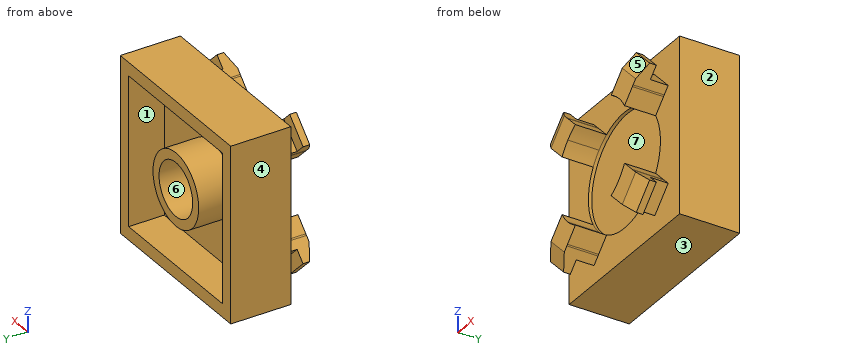
from build123d import *

# Parameters (mm, degrees)
SKETCH2_W            = 15.8
SKETCH2_H            = 15.8
BOSS_EXTRUDE2_DEPTH  = 5.4
SKETCH4_W            = 13.4
SKETCH4_H            = 13.4
CUT_EXTRUDE1_DEPTH   = 3.2
SKETCH7_R            = 3.265
SKETCH7_R_2          = 2.4
BOSS_EXTRUDE5_DEPTH  = 3.2
SKETCH8_R            = 5.15
CUT_EXTRUDE2_DEPTH   = 0.3
BOSS_EXTRUDE8_DEPTH  = 2.8
SKETCH27_W           = 2.7
SKETCH27_H           = 1.2
BOSS_EXTRUDE10_DEPTH = 1.2
CUT_EXTRUDE3_DEPTH   = 2.7
CIRPATTERN1_COUNT    = 4


with BuildPart() as part:
    # Sketch2 → Boss-Extrude2 (new body)
    with BuildSketch(Plane(origin=(0, 0, 0), x_dir=(1, 0, 0), z_dir=(0, 1, 0))):
        with Locations((7.9, 7.9)):
            Rectangle(SKETCH2_W, SKETCH2_H)
    extrude(amount=-BOSS_EXTRUDE2_DEPTH)

    # Sketch4 → Cut-Extrude1 (cut)
    with BuildSketch(Plane(origin=(0, 0, 0), x_dir=(1, 0, 0), z_dir=(0, 1, 0))):
        with Locations((7.9, 7.9)):
            Rectangle(SKETCH4_W, SKETCH4_H)
    extrude(amount=-CUT_EXTRUDE1_DEPTH, mode=Mode.SUBTRACT)

    # Sketch7 → Boss-Extrude5 (add)
    with BuildSketch(Plane(origin=(0, -3.2, 0), x_dir=(1, 0, 0), z_dir=(0, 1, 0))):
        with Locations((7.85, 7.85)):
            Circle(SKETCH7_R)
        with Locations((7.85, 7.85)):
            Circle(SKETCH7_R_2, mode=Mode.SUBTRACT)
    extrude(amount=BOSS_EXTRUDE5_DEPTH)

    # Sketch8 → Cut-Extrude2 (cut)
    with BuildSketch(Plane(origin=(0, -5.4, 0), x_dir=(-1, 0, 0), z_dir=(0, -1, 0))):
        with Locations((-7.9, 7.9)):
            Circle(SKETCH8_R)
    extrude(amount=-CUT_EXTRUDE2_DEPTH, mode=Mode.SUBTRACT)

    # Sketch11 → Boss-Extrude8 (add)
    with BuildSketch(Plane.XZ.offset(5.4)):
        Polygon((11.683021279, -2.207790411), (12.637615434, -3.162384566), (13.203300859, -2.596699141), (12.248706704, -1.642104986), align=None)
        with BuildLine():
            ThreePointArc((11.585853022, -2.304958669), (12.133497372, -2.706975833), (12.637615434, -3.162384566))
            Line((12.637615434, -3.162384566), (11.683021279, -2.207790411))
            Line((11.683021279, -2.207790411), (11.585853022, -2.304958669))
        make_face()
        with BuildLine():
            ThreePointArc((10.459662524, -3.431149167), (11.028098464, -3.808851017), (11.541599923, -4.258400077))
            Line((11.541599923, -4.258400077), (12.637615434, -3.162384566))
            ThreePointArc((12.637615434, -3.162384566), (12.133497372, -2.706975833), (11.585853022, -2.304958669))
            Line((11.585853022, -2.304958669), (10.459662524, -3.431149167))
        make_face()
        with BuildLine():
            Line((12.637615434, -3.162384566), (11.541599923, -4.258400077))
            ThreePointArc((11.541599923, -4.258400077), (11.991148983, -4.771901536), (12.368850833, -5.340337476))
            Line((12.368850833, -5.340337476), (13.495041331, -4.214146978))
            ThreePointArc((13.495041331, -4.214146978), (13.093024167, -3.666502628), (12.637615434, -3.162384566))
        make_face()
        with BuildLine():
            Line((13.592209589, -4.116978721), (12.637615434, -3.162384566))
            ThreePointArc((12.637615434, -3.162384566), (13.093024167, -3.666502628), (13.495041331, -4.214146978))
            Line((13.495041331, -4.214146978), (13.592209589, -4.116978721))
        make_face()
        Polygon((13.203300859, -2.596699141), (12.637615434, -3.162384566), (13.592209589, -4.116978721), (14.157895014, -3.551293296), align=None)
    boss_extrude8 = extrude(amount=BOSS_EXTRUDE8_DEPTH)

    # Sketch27 → Boss-Extrude10 (add)
    with BuildSketch(Plane(origin=(5.303300859, 0, 5.303300859), x_dir=(0.707106781, 0, -0.707106781), z_dir=(0.707106781, 0, 0.707106781))):
        with Locations((11.172287143, -7.6)):
            Rectangle(SKETCH27_W, SKETCH27_H)
    boss_extrude10 = extrude(amount=BOSS_EXTRUDE10_DEPTH)

    # Sketch28 → Cut-Extrude3 (cut)
    with BuildSketch(Plane(origin=(6.945405845, 0, -6.945405845), x_dir=(0.707106781, 0, 0.707106781), z_dir=(-0.707106781, 0, 0.707106781))):
        Polygon((8.7, -7.6), (7.215606324, -8.2), (8.7, -8.2), align=None)
    cut_extrude3 = extrude(amount=-CUT_EXTRUDE3_DEPTH, mode=Mode.SUBTRACT)

    # CirPattern1: Boss-Extrude8, Boss-Extrude10, Cut-Extrude3 ×4 about axis
    cirpattern1_axis = Axis((7.9, 0, -7.9), (0, 1, 0))
    for i in range(1, CIRPATTERN1_COUNT):
        add(boss_extrude8.rotate(cirpattern1_axis, i * 360 / CIRPATTERN1_COUNT))
        add(boss_extrude10.rotate(cirpattern1_axis, i * 360 / CIRPATTERN1_COUNT))
        add(cut_extrude3.rotate(cirpattern1_axis, i * 360 / CIRPATTERN1_COUNT), mode=Mode.SUBTRACT)


solid = part.part
Geometry: final body of the model. Coordinates: model frame, mm. Face numbers are marked on the shaded views. A direction names the side the tool comes from. Give positions to 0.01 mm unless a question says otherwise; leave off trailing zeros. Write each loop counter-clockwise with the first axis right and the second up, starting at its lowest first coordinate (ties: lowest second). Pieces come first, ordered by that corner, then holes. Notation, with made-up numbers: (-21.75, -23.5) - (29.25, -23.5) arc R23 cw to (29.25, -4.5) - close; hole circle Ø3 at (60, -10.5). An arc over 180 degrees is marked (long way). Return JSON: item names as keys, results as strings. Group by question number.
1) Line query: line 1 (Z direction, x = 7.85, y = -1.25) (3 decimals); line 2 (X direction, y = -1.55, z = -7.85) (3 decimals); line 3 (X direction, y = -5.3, z = -7.9). Output: solid intervals per line, ascending.
2) Set-up query: the marked faces 5, 6 and 7. Return all of +Z, -Z, +X, -X, +Y, -Y with unobstructed straight access to the full face (end or side cutting, diameter ignored); none if empty.
3) Section C-C on x = 3. Return the cut outline in (y, z).
4) First-contact query: P1, Ø0.8, axis at x = 3, z = -13, coming from the +Y side; P2, Ø5, axis at x = 9, z = -6, coming from the -Y side; P3, Ø3, axis at x = 12.5, z = -7.5, coming from the -Y side. Flat tips, straight axial feed; report the tip coordinate or a pass-through.
5) Mould query, pull axis X, two halves, no side actions, for the marked faces 1, 2, 3 and 4. Classes: released by +X, released by -X, zero draft, split by the parting line, or undercut.
6) Section B-B on y = -6.75. Return the cut outline in (x, z).
7) Section A-A on y = -2.5. Return the cut outline in (x, z) (3 decimals), plus the area to 3 significant figures.
8) Section D-D on z = -7.25. Return the cut outline in (x, y), plus the area to 3 significant figures.
Filled in:
{
 "1": {"line 1": "z = -15.8 to -14.6, -11.115 to -10.25, -5.45 to -4.585, -1.2 to 0", "line 2": "x = 0 to 1.2, 4.585 to 5.45, 10.25 to 11.115, 14.6 to 15.8", "line 3": "x = 0 to 2.75, 13.05 to 15.8"},
 "2": {"face 5": "+Z, +X, -Y", "face 6": "+Y", "face 7": "-Y"},
 "3": {"outline": "(-8.2, -13.2) - (-7.77, -14.71) - (-7, -14.71) - (-7, -13.61) - (-5.4, -13.61) - (-5.4, -15.8) - (0, -15.8) - (0, -14.6) - (-3.2, -14.6) - (-3.2, -1.2) - (0, -1.2) - (0, 0) - (-5.4, 0) - (-5.4, -2.19) - (-7, -2.19) - (-7, -1.09) - (-7.77, -1.09) - (-8.2, -2.6) - (-8.2, -4.91) - (-5.4, -4.91) - (-5.4, -6.31) - (-5.1, -6.31) - (-5.1, -9.49) - (-5.4, -9.49) - (-5.4, -10.89) - (-8.2, -10.89) - close"},
 "4": {"P1": "stops at y = -3.2", "P2": "stops at y = -5.1", "P3": "stops at y = -5.4"},
 "5": {"face 1": "undercut", "face 2": "released by +X", "face 3": "zero draft", "face 4": "released by -X"},
 "6": {"outline": "(1.64, -12.25) - (3.55, -14.16) - (5.34, -12.37) arc R5.15 cw to (3.43, -10.46) - close; (1.64, -3.55) - (3.43, -5.34) arc R5.15 cw to (5.34, -3.43) - (3.55, -1.64) - close; (10.46, -12.37) - (12.25, -14.16) - (14.16, -12.25) - (12.37, -10.46) arc R5.15 cw to start; (10.46, -3.43) arc R5.15 cw to (12.37, -5.34) - (14.16, -3.55) - (12.25, -1.64) - close"},
 "7": {"outline": "(0, -15.8) - (15.8, -15.8) - (15.8, 0) - (0, 0) - close; circle Ø6.53 at (7.85, -7.85); hole (1.2, -14.6) - (14.6, -14.6) - (14.6, -1.2) - (1.2, -1.2) - close; hole circle Ø4.8 at (7.85, -7.85)", "area": "85.5 mm^2"},
 "8": {"outline": "(0, -5.4) - (2.79, -5.4) - (2.79, -5.1) - (13.01, -5.1) - (13.01, -5.4) - (15.8, -5.4) - (15.8, 0) - (14.6, 0) - (14.6, -3.2) - (11.06, -3.2) - (11.06, 0) - (10.17, 0) - (10.17, -3.2) - (5.53, -3.2) - (5.53, 0) - (4.64, 0) - (4.64, -3.2) - (1.2, -3.2) - (1.2, 0) - (0, 0) - close", "area": "45.0 mm^2"}
}
